Can you work these out from the model? Positions are in its coordinate system, mm. A direction names the side the tool comes from. Give positions to 0.01 mm unless a question says otherwise; leave off trailing zeros. Order: outer loops, then holes, each group sorted by start corner. A loop starts at its lowest first (then second) coordinate and runs counter-clockwise, first axis right, second up. Notation, with made-up numbers: (-26.5, 42) - (13.5, 42) arc R4 ccw to (13.5, 49) - close; hole circle Ø6 at (46.5, 51). An arc over 180 degrees is marked (long way). Use one line per item in the form item = value. Start each with the question number.
1) We'd pull the mould along Z, two halves only. Please class faces 3 (the flat face through (-1, 76.2, 8)), 4 (the cylindrical face through (32.417, -1.067, 0.025)), 5 (the flat face through (57.15, -4, 22)): released by +Z, released by -Z, zero draft, split by the parting line, or undercut.
2) Which directions (+Z, -Z, +X, -X, +Y, -Y) give clear straight access to the entire face, cutting with the end or side of a thin tool? Please do faces 1 (the flat face through (63.5, -1, 22)), 2 (the flat face through (-1, -4, 25.4)).
3) Suppose I cut it at C-C, the plane z = -12. Write out the boundary of the cut face in (x, y).
4) Suppose I cut it at A-A, the plane y = 6. Write out the boundary of the cut face in (x, z).
5) Suppose I cut it at B-B, the plane x = 9.5. Write out the boundary of the cut face in (y, z), and give its area (3 significant figures).
6) For pin 1 (8 mm diameter, centred on y = -6.5, z = -9.5, fed in from -X); pin 2 (2 mm diameter, centred on y = -9, z = -5, fed in from -X); pin 3 (1.5 mm diameter, centred on y = -50, z = 6.5, fed in from +X), each with a flat end and sliding along its axis, tell me the tip position at first contact or that it passes through.
7) Please list where these lines run through material, in increasing order: probe 1 along Z at (x, y) = (-6.5, -55); probe 2 along X at (y, z) = (0, 24); probe 3 along Y at (x, z) = (19, 9).
```python
from build123d import *

# Parameters (mm, degrees)
F0_W     = 127
F0_H     = 63.5
F1_DEPTH = 76.2
F3_DEPTH = 152.4
F4_T     = -6.35


with BuildPart() as f1:
    # F0 (on Front) → F1 (new body, symmetric)
    with BuildSketch(Plane.XZ):
        Rectangle(F0_W, F0_H)
    extrude(amount=F1_DEPTH, both=True)

    # F2 (on face) → F3 (cut, through all)
    with BuildSketch(Plane.XZ.offset(76.2)):
        with BuildLine():
            Line((63.5, -31.75), (63.5, 12.7))
            ThreePointArc((63.5, 12.7), (32.069104, -0.319104), (19.05, -31.75))
            Line((19.05, -31.75), (63.5, -31.75))
        make_face()
        with BuildLine():
            ThreePointArc((-19.05, -31.75), (-32.069104, -0.319104), (-63.5, 12.7))
            Line((-63.5, 12.7), (-63.5, -31.75))
            Line((-63.5, -31.75), (-19.05, -31.75))
        make_face()
    extrude(amount=-F3_DEPTH, mode=Mode.SUBTRACT)

    # F4
    f4_openings = [f1.faces().sort_by_distance(p)[0] for p in [
        (0, -76.2, 8.06084),
    ]]
    offset(amount=F4_T, openings=f4_openings)


solid = f1.part
```
Result sheet:
q1.face_3 = zero draft
q1.face_4 = released by -Z
q1.face_5 = undercut
q2.face_1 = +Z, -Z, +X, +Y, -Y
q2.face_2 = -Y
q3.outline = (-23.68, -76.2) - (-16.7, -76.2) - (-16.7, 69.85) - (16.7, 69.85) - (16.7, -76.2) - (23.68, -76.2) - (23.68, 76.2) - (-23.68, 76.2) - close
q4.outline = (-63.5, 12.7) arc R44.45 cw to (-19.05, -31.75) - (19.05, -31.75) arc R44.45 cw to (63.5, 12.7) - (63.5, 31.75) - (-63.5, 31.75) - close; hole (-57.15, 18.65) arc R50.8 cw to (-13.1, -25.4) - (13.1, -25.4) arc R50.8 cw to (57.15, 18.65) - (57.15, 25.4) - (-57.15, 25.4) - close
q5.outline = (-76.2, -31.75) - (76.2, -31.75) - (76.2, 31.75) - (-76.2, 31.75) - (-76.2, 25.4) - (69.85, 25.4) - (69.85, -25.4) - (-76.2, -25.4) - close
q5.area = 2,260 mm²
q6.pin_1 = -27.63
q6.pin_2 = -28.78
q6.pin_3 = 42.17
q7.probe_1 = -31.75 to -25.4, 25.4 to 31.75
q7.probe_2 = -63.5 to -57.15, 57.15 to 63.5
q7.probe_3 = 69.85 to 76.2
